Can you work these out from the model? Positions are in its coordinate system, mm. A direction names the side the tool comes from. Coordinates: 2 decimals unless noted, no trailing zeros. Loops run counter-clockwise (first coordinate to the right, second up) from the corner with the lowest first, then second, coordinate; pieces in that order, holes last. Notation, with made-up numbers: M -11.5,-35.5 L 36.5,-35.5 A23 ccw 36.5,-19.5 Z; hole C -10,22.5 d10. An arc over 180 degrees is marked long. Answer as a JSON object with one key per item and string values. Group by question number.
Item 1: If I drill on line 1 (X direction, y = 1.85, z = 0); line 2 (Z direction, x = -53, y = 1.95) (3 decimals); line 3 (Z direction, x = 40.09, y = 1.7), over which ranges is the centre line in solid material (lowest first)?
Item 2: We'd pull the mould along X, two halves only. Please class faces 5 (the flat face through (0, 32.5, 0)), 6 (the flat face through (30, 4, 0)), 7 (the flat face through (-59, 2, 0)): +X half, -X half, draft (parallel to the pull), parting line (faces both ways), or undercut.
Item 3: Suppose I cut it at D-D (x = -17). Write out the boundary of the cut face in (y, z).
Item 4: I'm going to push flat-ended pins straight in: pin 1 Ø0.5 at (x, z) = (-6, -4.5) entering from +Y; pin 2 Ø2.5 at (x, z) = (53, 5) entering from -Y; pin 3 Ø1.5 at (y, z) = (22, -12) entering from +X; pin 4 Ø18 at (x, z) = (-43.5, 1.5) entering from +Y. Where does each tip first touch, or does it pass through?
Item 5: Suppose I cut it at A-A (x = 40.09). Write out the boundary of the cut face in (y, z).
Item 6: Suppose I cut it at C-C (z = 0). Write out the boundary of the cut face in (x, y).
Item 7: Suppose I cut it at B-B (y = 26). Write out the boundary of the cut face in (x, z) (3 decimals), then the cut area to 3 significant figures.
Item 8: Which directions (+Z, -Z, +X, -X, +Y, -Y) give clear straight access to the entire face, cutting with the end or side of a thin tool? Please do faces 1 (the flat face through (-26, 4, 0)), 2 (the flat face through (40, 5, -12)), 3 (the cylindrical face through (58.248, 2.465, -17.287)), 4 (the flat face through (-40, 5, -12)).
```python
from build123d import *

# Parameters (mm, degrees)
SKETCH1_W            = 20
SKETCH1_H            = 36
BOSS_EXTRUDE1_DEPTH  = 4
SKETCH2_W            = 20
SKETCH2_H            = 36
BOSS_EXTRUDE2_DEPTH  = 28.5
BOSS_EXTRUDE3_DEPTH  = 1
FILLET1_R            = 0.7
FILLET3_R            = 0.7
FILLET3_OF_MIRROR3_R = 0.7
FILLET4_R            = 0.7
SKETCH14_R           = 0.875
CUT_EXTRUDE3_DEPTH   = 68.537026882
SKETCH16_R           = 7.5
CUT_EXTRUDE4_DEPTH   = 10
SKETCH18_R           = 0.875
CUT_EXTRUDE5_DEPTH   = 10


with BuildPart() as part:
    # Sketch1 → Boss-Extrude1 (new body)
    with BuildSketch(Plane(origin=(0, 0, 0), x_dir=(1, 0, 0), z_dir=(0, 1, 0))):
        with BuildLine():
            Line((-10, -18), (-10, 18))
            Line((-10, 18), (-56.5, 18))
            ThreePointArc((-56.5, 18), (-58.267766953, 17.267766953), (-59, 15.5))
            Line((-59, 15.5), (-59, -15.5))
            ThreePointArc((-59, -15.5), (-58.267766953, -17.267766953), (-56.5, -18))
            Line((-56.5, -18), (-10, -18))
        make_face()
        Rectangle(SKETCH1_W, SKETCH1_H)
        with BuildLine():
            ThreePointArc((59, 15.5), (58.267766953, 17.267766953), (56.5, 18))
            Line((56.5, 18), (10, 18))
            Line((10, 18), (10, -18))
            Line((10, -18), (56.5, -18))
            ThreePointArc((56.5, -18), (58.267766953, -17.267766953), (59, -15.5))
            Line((59, -15.5), (59, 15.5))
        make_face()
    extrude(amount=BOSS_EXTRUDE1_DEPTH)

    # Sketch2 → Boss-Extrude2 (add)
    with BuildSketch(Plane(origin=(0, 4, 0), x_dir=(1, 0, 0), z_dir=(0, 1, 0))):
        Rectangle(SKETCH2_W, SKETCH2_H)
    extrude(amount=BOSS_EXTRUDE2_DEPTH)

    # Sketch7 → Boss-Extrude3 (add)
    with BuildSketch(Plane(origin=(0, 4, 0), x_dir=(1, 0, 0), z_dir=(0, 1, 0))):
        with BuildLine():
            Line((-51, 11), (-10, 11))
            Line((-10, 11), (-10, 18))
            Line((-10, 18), (-56.5, 18))
            ThreePointArc((-56.5, 18), (-58.267766953, 17.267766953), (-59, 15.5))
            Line((-59, 15.5), (-59, -15.5))
            ThreePointArc((-59, -15.5), (-58.267766953, -17.267766953), (-56.5, -18))
            Line((-56.5, -18), (-10, -18))
            Line((-10, -18), (-10, -11))
            Line((-10, -11), (-51, -11))
            Line((-51, -11), (-51, 11))
        make_face()
    boss_extrude3 = extrude(amount=BOSS_EXTRUDE3_DEPTH)

    # Fillet1
    fillet1_edges = [part.edges().sort_by_distance(p)[0] for p in [
        (-51, 4.5, -11),
    ]]
    fillet(fillet1_edges, radius=FILLET1_R)

    # Fillet3
    fillet3_edges = [part.edges().sort_by_distance(p)[0] for p in [
        (-51, 4.5, 11),
    ]]
    fillet(fillet3_edges, radius=FILLET3_R)

    # Mirror3: Boss-Extrude3 across plane
    add(boss_extrude3.mirror(Plane(origin=(0, 0, 0), x_dir=(0, 0, 1), z_dir=(1, 0, 0))))

    # Fillet3 of Mirror3
    fillet3_of_mirror3_edges = [part.edges().sort_by_distance(p)[0] for p in [
        (51, 4.5, 11),
    ]]
    fillet(fillet3_of_mirror3_edges, radius=FILLET3_OF_MIRROR3_R)

    # Fillet4
    fillet4_edges = [part.edges().sort_by_distance(p)[0] for p in [
        (51, 4.5, -11),
    ]]
    fillet(fillet4_edges, radius=FILLET4_R)

    # Sketch14 → Cut-Extrude3 (cut, through all)
    with BuildSketch(Plane(origin=(0, 5, 0), x_dir=(1, 0, 0), z_dir=(0, 1, 0))):
        with Locations(Location((-53, -5, 0), (0, 0, 270))):
            Circle(SKETCH14_R)
        with Locations(Location((-53, 5, 0), (0, 0, 270))):
            Circle(SKETCH14_R)
        with Locations(Location((53, -5, 0), (0, 0, 90))):
            Circle(SKETCH14_R)
        with Locations(Location((53, 5, 0), (0, 0, 90))):
            Circle(SKETCH14_R)
    extrude(amount=-CUT_EXTRUDE3_DEPTH, mode=Mode.SUBTRACT)

    # Sketch16 → Cut-Extrude4 (cut)
    with BuildSketch(Plane.XZ):
        with Locations(Location((-40.09, 0, 0), (0, 0, 270))):
            Circle(SKETCH16_R)
    cut_extrude4 = extrude(amount=-CUT_EXTRUDE4_DEPTH, mode=Mode.SUBTRACT)

    # Mirror4: Cut-Extrude4 across plane
    add(cut_extrude4.mirror(Plane.ZY), mode=Mode.SUBTRACT)

    # Sketch18 → Cut-Extrude5 (cut)
    with BuildSketch(Plane(origin=(0, 32.5, 0), x_dir=(1, 0, 0), z_dir=(0, 1, 0))):
        with Locations(Location((-6, -5, 0), (0, 0, 270))):
            Circle(SKETCH18_R)
        with Locations(Location((-6, 5, 0), (0, 0, 270))):
            Circle(SKETCH18_R)
        with Locations(Location((6, 5, 0), (0, 0, 270))):
            Circle(SKETCH18_R)
        with Locations(Location((6, -5, 0), (0, 0, 270))):
            Circle(SKETCH18_R)
    extrude(amount=-CUT_EXTRUDE5_DEPTH, mode=Mode.SUBTRACT)


solid = part.part
```
From the geometry:
{
 "1": {"line 1": "-59 to -47.59, -32.59 to 32.59, 47.59 to 59", "line 2": "-18 to -5.875, -4.125 to 4.125, 5.875 to 18", "line 3": "-18 to -7.5, 7.5 to 18"},
 "2": {"face 5": "draft", "face 6": "undercut", "face 7": "-X half"},
 "3": {"outline": "M 0,-18 L 5,-18 L 5,-11 L 4,-11 L 4,11 L 5,11 L 5,18 L 0,18 Z"},
 "4": {"pin 1": "y = 22.5", "pin 2": "y = 0", "pin 3": "x = 10", "pin 4": "y = 5"},
 "5": {"outline": "M 0,-18 L 5,-18 L 5,-11 L 4,-11 L 4,-7.5 L 0,-7.5 Z; M 0,7.5 L 4,7.5 L 4,11 L 5,11 L 5,18 L 0,18 Z"},
 "6": {"outline": "M -59,0 L -47.59,0 L -47.59,4 L -51,4 L -51,5 L -59,5 Z; M -32.59,0 L 32.59,0 L 32.59,4 L 10,4 L 10,32.5 L -10,32.5 L -10,4 L -32.59,4 Z; M 47.59,0 L 59,0 L 59,5 L 51,5 L 51,4 L 47.59,4 Z"},
 "7": {"outline": "M -10,-18 L 10,-18 L 10,18 L -10,18 Z; hole C -6,-5 d1.75; hole C -6,5 d1.75; hole C 6,-5 d1.75; hole C 6,5 d1.75", "area": "710 mm2"},
 "8": {"face 1": "+Y", "face 2": "+Z, -Z, +X, +Y", "face 3": "-Z, +X, +Y, -Y", "face 4": "+Z, -Z, -X, +Y"}
}
